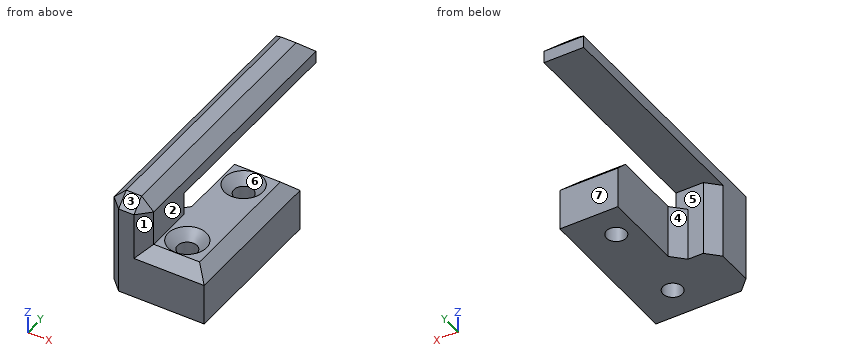
from build123d import *

# Parameters (mm, degrees)
SKETCH1_R                       = 1.6
BOSS_EXTRUDE1_DEPTH             = 8.8
SKETCH2_W                       = 6.5
SKETCH2_H                       = 10
BOSS_EXTRUDE2_DEPTH             = 3.7
BOSS_EXTRUDE2_DIRECTION_2_REACH = 30.332
SKETCH3_W                       = 6.5
SKETCH3_H                       = 44.6
BOSS_EXTRUDE3_DEPTH             = 4
SKETCH4_W                       = 6.5
SKETCH4_H                       = 44.6
CUT_EXTRUDE1_DEPTH              = 51.173797943
CHAMFER2_SIZE                   = 2
CHAMFER3_SIZE                   = 1.55


with BuildPart() as part:
    # Sketch1 → Boss-Extrude1 (new body)
    with BuildSketch(Plane.XY):
        Polygon((0, 0), (8, 0), (9.5, 0), (9.5, 25.2), (8, 25.2), (0, 25.2), align=None)
        with Locations((3.5, 20)):
            Circle(SKETCH1_R, mode=Mode.SUBTRACT)
        with Locations(Location((3.5, 5.2, 0), (0, 0, 180))):
            Circle(SKETCH1_R, mode=Mode.SUBTRACT)
    extrude(amount=BOSS_EXTRUDE1_DEPTH)

    # Sketch2 → Boss-Extrude2 (add)
    with BuildSketch(Plane.XY.offset(8.8)):
        with Locations((12.75, 5)):
            Rectangle(SKETCH2_W, SKETCH2_H)
    boss_extrude2 = extrude(amount=BOSS_EXTRUDE2_DEPTH)

    # Boss-Extrude2 direction 2: up to this face of the body (flat: up to its plane)
    boss_extrude2_direction_2_end = Plane(part.part.faces().sort_by_distance((4.840035102, 12.6, 0))[0])
    # Sketch2 → Boss-Extrude2 direction 2 (add, up to the picked face)
    with BuildSketch(Plane.XY.offset(8.8), mode=Mode.PRIVATE) as boss_extrude2_direction_2_sk1:
        with Locations((12.75, 5)):
            Rectangle(SKETCH2_W, SKETCH2_H)
    boss_extrude2_direction_2_tool1 = split(extrude(boss_extrude2_direction_2_sk1.sketch, amount=-BOSS_EXTRUDE2_DIRECTION_2_REACH, mode=Mode.PRIVATE), bisect_by=boss_extrude2_direction_2_end, keep=Keep.BOTH, mode=Mode.PRIVATE)
    boss_extrude2_direction_2 = boss_extrude2_direction_2_tool1.solids().sort_by(Axis((12.75, 5, 8.8), (0, 0, -1)))[0]
    add(boss_extrude2_direction_2)

    # Sketch3 → Boss-Extrude3 (add)
    with BuildSketch(Plane.XY.offset(12.5)):
        with Locations((12.75, 22.3)):
            Rectangle(SKETCH3_W, SKETCH3_H)
    boss_extrude3 = extrude(amount=BOSS_EXTRUDE3_DEPTH)

    # Mirror1: Boss-Extrude2, Boss-Extrude2 direction 2, Boss-Extrude3 across plane
    add(boss_extrude2.mirror(Plane(origin=(4.75, 0, 0), x_dir=(0, 0, 1), z_dir=(1, 0, 0))))
    add(boss_extrude2_direction_2.mirror(Plane(origin=(4.75, 0, 0), x_dir=(0, 0, 1), z_dir=(1, 0, 0))))
    add(boss_extrude3.mirror(Plane(origin=(4.75, 0, 0), x_dir=(0, 0, 1), z_dir=(1, 0, 0))))

    # Sketch4 → Cut-Extrude1 (cut, through all)
    with BuildSketch(Plane.XY.offset(16.5)):
        with Locations((12.75, 22.3)):
            Rectangle(SKETCH4_W, SKETCH4_H)
    extrude(amount=-CUT_EXTRUDE1_DEPTH, mode=Mode.SUBTRACT)

    # Chamfer2
    chamfer2_edges = [part.edges().sort_by_distance(p)[0] for p in [
        (9.5, 12.6, 8.8),
        (4.75, 25.2, 8.8),
        (0, 10, 4.4),
        (0, 0, 12.65),
        (-6.5, 0, 8.25),
        (-6.5, 10, 6.25),
        (0, 22.3, 16.5),
        (-3.25, 44.6, 16.5),
        (-6.5, 22.3, 16.5),
        (-3.25, 0, 16.5),
        (4.75, 0, 8.8),
    ]]
    chamfer(chamfer2_edges, length=CHAMFER2_SIZE)

    # Chamfer3
    chamfer3_edges = [part.edges().sort_by_distance(p)[0] for p in [
        (1.9, 20, 8.8),
        (5.1, 5.2, 8.8),
    ]]
    chamfer(chamfer3_edges, length=CHAMFER3_SIZE)


solid = part.part
For this review, take the finished solid that the model builds, in its own axes (mm). Face numbers are marked on the shaded views. A direction names the side the tool comes from. Round coordinates to 2 decimals unless told otherwise and drop trailing zeros. Loops run counter-clockwise (first coordinate to the right, second up) from the corner with the lowest first, then second, coordinate; pieces in that order, holes last. Notation, with made-up numbers: (51.25, 85) - (94.25, 85) arc R27 ccw to (94.25, 107) - close; hole circle Ø7 at (56.25, 53). An arc over 180 degrees is marked (long way). Use one line per item in the form item = value.
Item 1: Clearance check with flat-ended pins moving along their axes: P1, Ø6, axis at y = 31, z = 11.5, coming from the +X side; P2, Ø2.5, axis at x = 3.5, y = 5.2, coming from the +Z side; P3, Ø5.5, axis at x = 4.5, z = 4.5, coming from the +Y side; P4, Ø7, axis at x = -4.5, y = 25.5, coming from the -Z side. State where each tip first meets the part, or that it passes through.
Answers:
P1 = 0
P2 = through
P3 = 25.2
P4 = 12.5
Item 2: Consider section A-A on y = 20. Write out the cut boundary in (x, z), then the cut area to 3 significant figures.
Answers:
outline = (-6.5, 12.5) - (0, 12.5) - (0, 14.5) - (-2, 16.5) - (-4.5, 16.5) - (-6.5, 14.5) - close; (0, 0) - (1.9, 0) - (1.9, 7.25) - (0.35, 8.8) - (0, 8.8) - close; (5.1, 0) - (9.5, 0) - (9.5, 6.8) - (7.5, 8.8) - (6.65, 8.8) - (5.1, 7.25) - close
area = 73.0 mm^2
Item 3: For line 1 (Y direction, x = 3.5, z = 5.75); line 2 (X direction, y = 5.2, z = 5.5); line 3 (Y direction, x = -3.5, z = 11.5), list the stretches that pass through material, from the lowest coordinate up.
Answers:
line_1 = 0 to 3.6, 6.8 to 18.4, 21.6 to 25.2
line_2 = -6.5 to 1.9, 5.1 to 9.5
line_3 = 0 to 10
Item 4: Consider section B-B on x = 3.5. Write out the cut boundary in (y, z).
Answers:
outline = (0, 0) - (3.6, 0) - (3.6, 7.25) - (2.05, 8.8) - (2, 8.8) - (0, 6.8) - close; (6.8, 0) - (18.4, 0) - (18.4, 7.25) - (16.85, 8.8) - (8.35, 8.8) - (6.8, 7.25) - close; (21.6, 0) - (25.2, 0) - (25.2, 6.8) - (23.2, 8.8) - (23.15, 8.8) - (21.6, 7.25) - close
Item 5: Consider section C-C on z = 6.25. Write out the cut boundary in (x, y).
Answers:
outline = (-6.5, 2) - (-4.5, 0) - (9.5, 0) - (9.5, 25.2) - (0, 25.2) - (0, 12) - (-2, 10) - (-4.5, 10) - (-6.5, 8) - close; hole circle Ø3.2 at (3.5, 5.2); hole circle Ø3.2 at (3.5, 20)
Item 6: Mouldability with a two-part tool opening along Z and no side actions: class the marked faces 5, 6 and 7 as +Z half, -Z half, draft (parallel to the pull), parting line (faces both ways), or undercut.
Answers:
face_5 = undercut
face_6 = +Z half
face_7 = draft
Item 7: Tool access review of the marked faces 1, 2, 3 and 4: name each direction out of +Z, -Z, +X, -X, +Y, -Y from which nothing blocks a thin tool from reaching the whole face with its end or side.
Answers:
face_1 = +Z, +X, -Y
face_2 = +Z, +X, +Y, -Y
face_3 = +Z, +X, -X, -Y
face_4 = -Z, -X, +Y
Item 8: Consider section D-D on z = 9.75. Write out the cut boundary in (x, y).
Answers:
outline = (-6.5, 2) - (-4.5, 0) - (-2, 0) - (0, 2) - (0, 10) - (-4.5, 10) - (-6.5, 8) - close
